For this review, take the finished solid that the model builds, in its own axes (mm). A direction names the side the tool comes from. Give positions to 0.01 mm unless a question says otherwise; leave off trailing zeros. Loops run counter-clockwise (first coordinate to the right, second up) from the corner with the lowest first, then second, coordinate; pieces in that order, holes last.
Autodesk Inventor part; units mm, degrees
ref_plane "YZ Plane" through (0, 0, 0) normal (1, 0, 0) x (0, 1, 0)
ref_plane "XZ Plane" through (0, 0, 0) normal (0, 1, 0) x (-1, 0, 0)
ref_plane "XY Plane" through (0, 0, 0) normal (0, 0, 1) x (1, 0, 0)
sketch "Sketch1" plane through (0, 0, 0) normal (0, 0, 1) x (1, 0, 0)
  line L0 (0, 12.3846) -> (17.8016, 12.3846)
  line L1 (17.8016, 12.3846) -> (17.8016, 0.6334)
  line L2 (17.8016, 0.6334) -> (0, 0.6334)
  line L3 (0, 0.6334) -> (0, 12.3846)
  point P0 (0, 0)
extrude "Extrusion1" add sketch "Sketch1" along normal blind 1.5
shell "Shell1" thickness 0.4 removed faces 1 at (5.9339, 8.4676, 0)
properties part number "a4"
Item 1: For L1, parallel to X at y = 7, z = 1; L2, parallel to Y at x = 9.75, z = 0.5; L3, parallel to Z at x = 8.75, y = 11, list the stretches that pass through material, from the lowest coordinate up.
Answer:
L1: x = 0 to 0.4, 17.4 to 17.8
L2: y = 0.63 to 1.03, 11.98 to 12.38
L3: z = 1.1 to 1.5
Item 2: Take a section at B-B on y = 4.75. Give the boundary of the cut face in (x, z).
Answer:
outline: (0, 0) - (0.4, 0) - (0.4, 1.1) - (17.4, 1.1) - (17.4, 0) - (17.8, 0) - (17.8, 1.5) - (0, 1.5) - close
Item 3: Clearance check with a flat-ended pin moving along its axis: pin 1 Ø1.5 at (x, y) = (16, 8.5) entering from -Z. State where the tip first meets the part, or that it passes through.
Answer:
pin 1: stops at z = 1.1
Item 4: Tool access review of faces 4 (the flat face through (8.8, 11.985, 0.5)), 5 (the flat face through (9, 12.385, 1)): name each direction out of +Z, -Z, +X, -X, +Y, -Y from which nothing blocks a thin tool from reaching the whole face with its end or side.
Answer:
face 4: -Z
face 5: +Z, -Z, +X, -X, +Y
Item 5: Take a section at C-C on x = 6.25. Give the boundary of the cut face in (y, z).
Answer:
outline: (0.63, 0) - (1.03, 0) - (1.03, 1.1) - (11.98, 1.1) - (11.98, 0) - (12.38, 0) - (12.38, 1.5) - (0.63, 1.5) - close
Item 6: The part is to be moulded in two halves that separate along Y. For faces 1 (the flat face through (9, 1.033, 0.5)), 2 (the flat face through (8.2, 0.88, 0)), 3 (the flat face through (9, 0.633, 1)), say which applies: released by +Y, released by -Y, zero draft, split by the parting line, or undercut.
Answer:
face 1: undercut
face 2: zero draft
face 3: released by -Y
Item 7: Take a section at A-A on z = 0.65. Give the boundary of the cut face in (x, y), and give its area (3 significant figures).
Answer:
outline: (0, 0.63) - (17.8, 0.63) - (17.8, 12.38) - (0, 12.38) - close; hole (0.4, 1.03) - (17.4, 1.03) - (17.4, 11.98) - (0.4, 11.98) - close
area: 23.0 mm2
